from build123d import *

# Parameters (mm, degrees)
BOSS_EXTRU_1_DEPTH      = 200
CHANFREIN1_SIZE2        = 3.618684617
CHANFREIN1_SIZE         = 3
CHANFREIN1_EDGE_2_SIZE2 = 3
CHANFREIN1_EDGE_2_SIZE  = 3.618684617
CONG_2_R                = 3


with BuildPart() as part:
    # Esquisse1 → Boss.-Extru.1 (new body)
    with BuildSketch(Plane.XY):
        with BuildLine():
            Line((-12.171180036, -17.570882511), (12.171180036, -17.570882511))
            Line((12.171180036, -17.570882511), (14.613263907, -2.343612169))
            ThreePointArc((14.613263907, -2.343612169), (13.502002072, 6.061018071), (7.960382718, 12.476870881))
            Line((7.960382718, 12.476870881), (6.669509845, 12.476870881))
            Line((6.669509845, 12.476870881), (6.669509845, 10.453594522))
            ThreePointArc((6.669509845, 10.453594522), (12.142715388, -2.512859527), (1.972784363, -12.242063627))
            ThreePointArc((1.972784363, -12.242063627), (0, -14.570882511), (-1.972784363, -12.242063627))
            ThreePointArc((-1.972784363, -12.242063627), (-12.142715388, -2.512859527), (-6.669509845, 10.453594522))
            Line((-6.669509845, 10.453594522), (-6.669509845, 12.476870881))
            Line((-6.669509845, 12.476870881), (-7.960382718, 12.476870881))
            ThreePointArc((-7.960382718, 12.476870881), (-13.502002072, 6.061018071), (-14.613263907, -2.343612169))
            Line((-14.613263907, -2.343612169), (-12.171180036, -17.570882511))
        make_face()
    extrude(amount=BOSS_EXTRU_1_DEPTH)

    # Chanfrein1
    chanfrein1_edges = [part.edges().sort_by_distance(p)[0] for p in [
        (12.171180036, -17.570882511, 100),
    ]]
    chamfer(chanfrein1_edges, length=CHANFREIN1_SIZE, length2=CHANFREIN1_SIZE2)

    # Chanfrein1 edge 2
    chanfrein1_edge_2_edges = [part.edges().sort_by_distance(p)[0] for p in [
        (-12.171180036, -17.570882511, 100),
    ]]
    chamfer(chanfrein1_edge_2_edges, length=CHANFREIN1_EDGE_2_SIZE, length2=CHANFREIN1_EDGE_2_SIZE2)

    # Congé2
    cong_2_edges = [part.edges().sort_by_distance(p)[0] for p in [
        (12.744206611, -13.997855937, 100),
        (-12.646236557, -14.608734422, 100),
    ]]
    fillet(cong_2_edges, radius=CONG_2_R)


solid = part.part
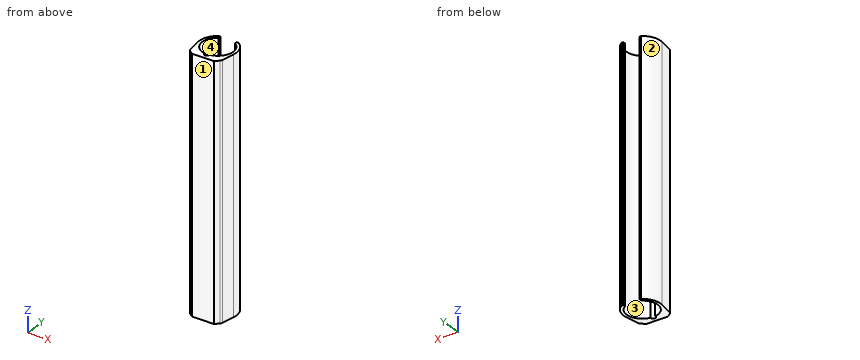
The listing builds one solid part. Answer for the finished solid, in the listing's coordinates (mm). Face numbers are marked on the shaded views. Coordinates: 2 decimals unless noted, no trailing zeros. Order: outer loops, then holes, each group sorted by start corner. A loop starts at its lowest first (then second) coordinate and runs counter-clockwise, first axis right, second up.
Q1. Consider line 1 (X direction, y = -10.5, z = 173); line 2 (Y direction, x = -8.25, z = 35); line 3 (X direction, y = 6, z = 163.5). Determine where each line is inside the solid, lowest interval first.
Q2. For a pull along X with two mould halves and no side action, classify the marked faces 1, 2, 3 and 4 as pulls with the +X half, pulls with the -X half, needs draft (parallel to the pull), parting line crosses it, or undercut.
Q3. A cutting plane is placed at C-C, the plane x = 0. Write down the section's boundary in (y, z).
Q4. A cutting plane is placed at B-B, the plane z = 118.5. Write down the section's boundary in (x, y), and give its area (3 significant figures).
Q5. A cutting plane is placed at A-A, the plane y = -6. Write down the section's boundary in (x, z), and give its area (3 significant figures).
Q6. Given P1, Ø1.6, axis at y = 11, z = 113, coming from the +X side; P2, Ø6, axis at y = -8.5, z = 174.5, coming from the +X side; P3, Ø2, axis at y = 11, z = 147.5, coming from the -X side, each flat-ended and moving along its own axis, determine where each tip first touches the part or whether it passes through.
Answers follow:
1. line 1: x = -13.31 to -6.6, 6.6 to 13.31
1. line 2: y = -17.57 to -9.26, 9.26 to 12.29
1. line 3: x = -13.53 to -10.85, 10.85 to 13.53
2. face 1: needs draft
2. face 2: pulls with the -X half
2. face 3: undercut
2. face 4: undercut
3. outline: (-17.57, 0) - (-14.57, 0) - (-14.57, 200) - (-17.57, 200) - close
4. outline: (-14.61, -2.34) - (-12.84, -13.38) arc R3 ccw to (-11.64, -15.34) - (-8.55, -17.57) - (9.17, -17.57) - (12.06, -14.68) arc R3 ccw to (12.9, -13.04) - (14.61, -2.34) arc R14.8 ccw to (7.96, 12.48) - (6.67, 12.48) - (6.67, 10.45) arc R12.4 cw to (1.97, -12.24) arc R2 cw (long way) to (-1.97, -12.24) arc R12.4 cw to (-6.67, 10.45) - (-6.67, 12.48) - (-7.96, 12.48) arc R14.8 ccw to start
4. area: 285 mm2
5. outline: (-14.03, 0) - (-10.85, 0) - (-10.85, 200) - (-14.03, 200) - close; (10.85, 0) - (14.03, 0) - (14.03, 200) - (10.85, 200) - close
5. area: 1,270 mm2
6. P1: stops at x = 10.72
6. P2: stops at x = 14.11
6. P3: stops at x = -10.91
